from build123d import *

# Parameters (mm, degrees)
SKETCH_1_R          = 2.5
EXTRUDE_1_DEPTH     = 40
CUT_EXTRUDE_1_REACH = 52.804
SKETCH_2_R          = 2.5
SKETCH_3_W          = 9
SKETCH_3_H          = 10
CUT_EXTRUDE_2_DEPTH = 20
FILLET_1_R          = 4
SKETCH_4_R          = 2.5
EXTRUDE_2_DEPTH     = 40


with BuildPart() as part:
    # 草图1 → 凸台-拉伸1 (new body)
    with BuildSketch(Plane(origin=(0, 0, 0), x_dir=(1, 0, 0), z_dir=(0, 1, 0))):
        with BuildLine():
            Line((0, -4.5), (30, -4.5))
            Line((30, -4.5), (30, -2.5))
            Line((30, -2.5), (3.741657387, -2.5))
            ThreePointArc((3.741657387, -2.5), (-2.121320344, 3.968626967), (0, -4.5))
        make_face()
        with Locations(Location((0, 0, 0), (0, 0, 270))):
            Circle(SKETCH_1_R, mode=Mode.SUBTRACT)
    extrude(amount=EXTRUDE_1_DEPTH)

    # 草图2 → 切除-拉伸1 (cut, up to next)
    with BuildSketch(Plane.XY.offset(4.5), mode=Mode.PRIVATE) as cut_extrude_1_sk1:
        with Locations((19.5, 30)):
            Circle(SKETCH_2_R)
    cut_extrude_1_tool1 = extrude(cut_extrude_1_sk1.sketch, amount=-CUT_EXTRUDE_1_REACH, mode=Mode.PRIVATE) & part.part
    # 草图2 → 切除-拉伸1 (cut, up to next)
    with BuildSketch(Plane.XY.offset(4.5), mode=Mode.PRIVATE) as cut_extrude_1_sk2:
        with Locations((19.5, 10)):
            Circle(SKETCH_2_R)
    cut_extrude_1_tool2 = extrude(cut_extrude_1_sk2.sketch, amount=-CUT_EXTRUDE_1_REACH, mode=Mode.PRIVATE) & part.part
    add(cut_extrude_1_tool1.solids().sort_by_distance((19.5, 30, 4.5))[0], mode=Mode.SUBTRACT)
    add(cut_extrude_1_tool2.solids().sort_by_distance((19.5, 10, 4.5))[0], mode=Mode.SUBTRACT)

    # 草图3 → 切除-拉伸2 (cut, symmetric)
    with BuildSketch(Plane(origin=(0, 0, 2.5), x_dir=(-1, 0, 0), z_dir=(0, 0, -1))):
        with Locations((0, 35)):
            Rectangle(SKETCH_3_W, SKETCH_3_H)
        with Locations((0, 15)):
            Rectangle(SKETCH_3_W, SKETCH_3_H)
    extrude(amount=CUT_EXTRUDE_2_DEPTH, both=True, mode=Mode.SUBTRACT)

    # 圆角1
    fillet_1_edges = [part.edges().sort_by_distance(p)[0] for p in [
        (30, 40, 3.5),
        (30, 0, 3.5),
    ]]
    fillet(fillet_1_edges, radius=FILLET_1_R)

    # 草图4 → 凸台-拉伸2 (add)
    with BuildSketch(Plane.XZ):
        with Locations(Location((0, 0, 0), (0, 0, 270))):
            Circle(SKETCH_4_R)
    extrude(amount=-EXTRUDE_2_DEPTH)


solid = part.part
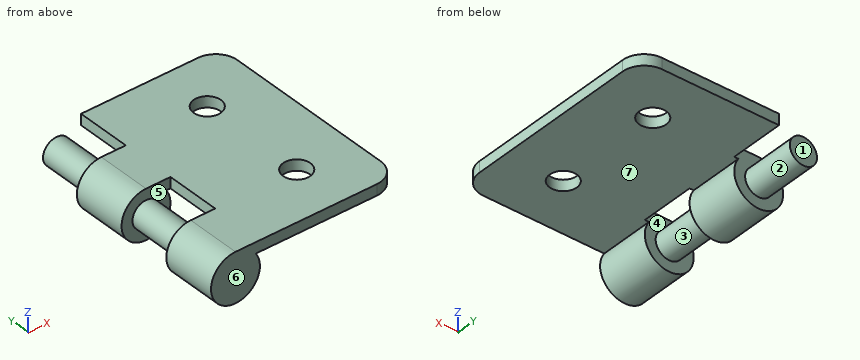
Verification items for the finished model (mm, model axes). Face numbers are marked on the shaded views. A direction names the side the tool comes from. Round coordinates to 2 decimals unless told otherwise and drop trailing zeros. Order: outer loops, then holes, each group sorted by start corner. A loop starts at its lowest first (then second) coordinate and runs counter-clockwise, first axis right, second up. Notation, with made-up numbers: (14.5, 57) -> (41.5, 57) arc R11 ccw to (41.5, 62) -> close; hole circle Ø10 at (84.25, 16.5). An arc over 180 degrees is marked (long way). Put each result on its own line as item: value.
1) Mould release check, pull along Y, two halves, no side actions. Record for the marked faces 4, 5, 6 and 7: +Y half, -Y half, draft (parallel to the pull), parting line (faces both ways), or undercut.
Final values:
face 4: undercut
face 5: undercut
face 6: -Y half
face 7: draft
2) Section check A-A (y = 32). Record the cut outline in (x, z).
Final values:
outline: circle Ø5 at (0, 0); (4.5, 2.5) -> (18, 2.5) -> (18, 4.5) -> (4.5, 4.5) -> close; (21, 2.5) -> (30, 2.5) -> (30, 4.5) -> (21, 4.5) -> close
3) Depth check by flat-ended pin: pin 1 (3 mm diameter, centred on x = 16, y = 12, fed in from -Z); pin 2 (1 mm diameter, centred on y = 27.5, z = -2.5, fed in from +X); pin 3 (2 mm diameter, centred on y = 14, z = 4, fed in from -X). Enter the tip coordinate at first touch or a pass-through.
Final values:
pin 1: stops at z = 2.5
pin 2: stops at x = 4.03
pin 3: stops at x = 4.5
4) Section check D-D (x = 20). Record the cut outline in (y, z).
Final values:
outline: (0, 2.5) -> (7.55, 2.5) -> (7.55, 4.5) -> (0, 4.5) -> close; (12.45, 2.5) -> (27.55, 2.5) -> (27.55, 4.5) -> (12.45, 4.5) -> close; (32.45, 2.5) -> (40, 2.5) -> (40, 4.5) -> (32.45, 4.5) -> close
5) Section check C-C (z = 0). Record the cut outline in (x, y).
Final values:
outline: (-4.5, 0) -> (4.5, 0) -> (4.5, 10) -> (2.5, 10) -> (2.5, 20) -> (4.5, 20) -> (4.5, 30) -> (2.5, 30) -> (2.5, 40) -> (-2.5, 40) -> (-2.5, 30) -> (-4.5, 30) -> (-4.5, 20) -> (-2.5, 20) -> (-2.5, 10) -> (-4.5, 10) -> close
6) Section check B-B (y = 28). Record the cut outline in (x, z), then the cut area to 3 significant figures.
Final values:
outline: (0, 4.5) arc R4.5 ccw (long way) to (3.74, 2.5) -> (18, 2.5) -> (18, 4.5) -> close; (21, 2.5) -> (30, 2.5) -> (30, 4.5) -> (21, 4.5) -> close
area: 112 mm^2
7) Material ranges on line 1 (Y direction, x = 19.5, z = 3.2); line 2 (Z direction, x = 27, y = 36.5); line 3 (Y direction, x = -0.5, z = -3.5), recorded low to high.
Final values:
line 1: y = 0 to 7.5, 12.5 to 27.5, 32.5 to 40
line 2: z = 2.5 to 4.5
line 3: y = 0 to 10, 20 to 30
8) Set-up check for the marked faces 1, 2 and 3: record each of +Z, -Z, +X, -X, +Y, -Y from which the full face is reachable in a straight line by a thin tool's end or side.
Final values:
face 1: +Z, -Z, +X, -X, +Y
face 2: +Y
face 3: none
